Geometry: final body of the model. Coordinates: model frame, mm. A direction names the side the tool comes from. Coordinates: 2 decimals unless noted, no trailing zeros. Write each loop counter-clockwise with the first axis right and the second up, starting at its lowest first coordinate (ties: lowest second). Pieces come first, ordered by that corner, then holes. Notation, with made-up numbers: M 40.5,22.25 L 81.5,22.25 A27 cw 81.5,61.25 Z; hole C 7,12.25 d1. An arc over 180 degrees is marked long. Write item = value, one per line. Start each with the question number.
Item 1: Section A-A on y = -5. Output: boundary loops of the cut face in (x, z).
Item 2: Pull-direction query (Z, two-part tool) for faces 4 (the flat face through (-10, 5, 5)), 5 (the cylindrical face through (-13.6, -4.93, 9.38)), 6 (the flat face through (-12, 2, 11.6)), 7 (the flat face through (-12, 0, 1.6)); classes: +Z half, -Z half, draft (parallel to the pull), parting line (faces both ways), or undercut.
Item 3: Ray query, L1, parallel to Y at x = -12, z = 10.5; L2, parallel to Y at x = -15.5, z = 2.75; L3, parallel to Z at x = -13.5, y = -6. Return the intervals inside material, ascending. Write a range as [from, to].
Item 4: Section B-B on x = -12. Output: boundary loops of the cut face in (y, z), plus the area to 3 significant figures.
Item 5: First-contact query: pin 1 Ø2 at (x, y) = (-12, -5.5) entering from +Z; pin 2 Ø3 at (x, y) = (-13, 0) entering from +Z. Flat tips, straight axial feed; report the tip coordinate or a pass-through.
Item 6: Section D-D on y = -0.5. Output: boundary loops of the cut face in (x, z), plus the area to 3 significant figures.
Item 7: Reachability of faces 1 (the cylindrical face through (-13.6, 0.07, 9.38)), 2 (the flat face through (-13, -3, 5)), 3 (the flat face through (-12, -7.5, 7)) from +Z, -Z, +X, -X, +Y, -Y: full face, straight path, thin tool, end or side. Return the list, or none.
Item 8: Section C-C on z = 8. Output: boundary loops of the cut face in (x, y), plus the area to 3 significant figures.
from build123d import *

# Parameters (mm, degrees)
SKETCH001_W     = 8
SKETCH001_H     = 15
PAD001_DEPTH    = 10
POCKET_DEPTH    = 16
SKETCH003_R     = 1.6
POCKET001_DEPTH = 5
SKETCH004_W     = 4
SKETCH004_H     = 5
POCKET002_DEPTH = 6


with BuildPart() as part:
    # Sketch001 (on Face1 of CopyPad) → Pad001 (new body)
    with BuildSketch(Plane.XY.offset(1.6)):
        with Locations((-12, 0)):
            Rectangle(SKETCH001_W, SKETCH001_H)
    extrude(amount=PAD001_DEPTH)

    # Sketch002 (on Face1 of Pad001) → Pocket (cut)
    with BuildSketch(Plane(origin=(0, -7.5, 1.6), x_dir=(1, 0, 0), z_dir=(0, -1, 0))):
        Polygon((-16, 10), (-16, 6), (-14.5, 10), align=None)
        Polygon((-8, 10), (-9.5, 10), (-8, 6), align=None)
    extrude(amount=-POCKET_DEPTH, mode=Mode.SUBTRACT)

    # Sketch003 (on Face5 of Pocket) → Pocket001 (cut)
    with BuildSketch(Plane.XY.offset(11.6)):
        with Locations((-12, 5)):
            Circle(SKETCH003_R)
        with Locations((-12, 0)):
            Circle(SKETCH003_R)
        with Locations((-12, -5)):
            Circle(SKETCH003_R)
    extrude(amount=-POCKET001_DEPTH, mode=Mode.SUBTRACT)

    # Sketch004 (on Face7 of Pocket001) → Pocket002 (cut)
    with BuildSketch(Plane(origin=(-16, 0, 1.6), x_dir=(0, -1, 0), z_dir=(-1, 0, 0))):
        with Locations((-5, 3)):
            Rectangle(SKETCH004_W, SKETCH004_H)
        with Locations((0, 3)):
            Rectangle(SKETCH004_W, SKETCH004_H)
        with Locations((5, 3)):
            Rectangle(SKETCH004_W, SKETCH004_H)
    extrude(amount=-POCKET002_DEPTH, mode=Mode.SUBTRACT)


solid = part.part
Responses:
q1.outline = M -16,1.6 L -8,1.6 L -8,7.6 L -9.5,11.6 L -10.4,11.6 L -10.4,7.1 L -10,7.1 L -10,2.1 L -16,2.1 Z; M -16,7.1 L -13.6,7.1 L -13.6,11.6 L -14.5,11.6 L -16,7.6 Z
q2.face_4 = undercut
q2.face_5 = draft
q2.face_6 = +Z half
q2.face_7 = -Z half
q3.L1 = [-7.5, -6.6], [-3.4, -1.6], [1.6, 3.4], [6.6, 7.5]
q3.L2 = [-7.5, -7], [-3, -2], [2, 3], [7, 7.5]
q3.L3 = [1.6, 2.1], [7.1, 11.6]
q4.outline = M -7.5,1.6 L 7.5,1.6 L 7.5,11.6 L 6.6,11.6 L 6.6,7.1 L 7,7.1 L 7,2.1 L 3,2.1 L 3,7.1 L 3.4,7.1 L 3.4,11.6 L 1.6,11.6 L 1.6,7.1 L 2,7.1 L 2,2.1 L -2,2.1 L -2,7.1 L -1.6,7.1 L -1.6,11.6 L -3.4,11.6 L -3.4,7.1 L -3,7.1 L -3,2.1 L -7,2.1 L -7,7.1 L -6.6,7.1 L -6.6,11.6 L -7.5,11.6 Z
q4.area = 46.8 mm²
q5.pin_1 = 2.1
q5.pin_2 = 11.6
q6.outline = M -16,1.6 L -8,1.6 L -8,7.6 L -9.5,11.6 L -10.48,11.6 L -10.48,7.1 L -10,7.1 L -10,2.1 L -16,2.1 Z; M -16,7.1 L -13.52,7.1 L -13.52,11.6 L -14.5,11.6 L -16,7.6 Z
q6.area = 30.3 mm²
q7.face_1 = +Z
q7.face_2 = -X
q7.face_3 = +Z, -Z, +X, -X, -Y
q8.outline = M -15.85,-7.5 L -8.15,-7.5 L -8.15,7.5 L -15.85,7.5 Z; hole C -12,-5 d3.2; hole C -12,0 d3.2; hole C -12,5 d3.2
q8.area = 91.4 mm²
